```python
from build123d import *

# Parameters (mm, degrees)
F0_W     = 34
F0_H     = 10
F1_DEPTH = 5


with BuildPart() as f1:
    # F0 (on Top) → F1 (new body)
    with BuildSketch(Plane.XY):
        with Locations((5, 0)):
            Rectangle(F0_W, F0_H)
        with BuildLine():
            ThreePointArc((-9.081139, -2.25), (-8.767748, 2.440352), (-4.75, 0))
            ThreePointArc((-4.75, 0), (-5.059648, -1.267748), (-5.918861, -2.25))
            ThreePointArc((-5.918861, -2.25), (-7.5, -2.75), (-9.081139, -2.25))
        make_face(mode=Mode.SUBTRACT)
        Polygon((-3.175426, 0), (-1.587713, 2.75), (1.587713, 2.75), (3.175426, 0), (1.587713, -2.75), (-1.587713, -2.75), align=None, mode=Mode.SUBTRACT)
        Polygon((5.247223, 0), (7.123612, 3.25), (10.876388, 3.25), (12.752777, 0), (10.876388, -3.25), (7.123612, -3.25), align=None, mode=Mode.SUBTRACT)
        Polygon((20.098076, 0), (18.799038, -2.25), (16.200962, -2.25), (14.901924, 0), (16.200962, 2.25), (18.799038, 2.25), align=None, mode=Mode.SUBTRACT)
        with BuildLine():
            Line((-5.918861, -2.25), (-9.081139, -2.25))
            ThreePointArc((-9.081139, -2.25), (-7.5, -2.75), (-5.918861, -2.25))
        make_face()
    extrude(amount=F1_DEPTH)


solid = f1.part
```
The model under review builds one solid part; all positions refer to its coordinate system, in mm. A direction names the side the tool comes from. Give positions to 0.01 mm unless a question says otherwise; leave off trailing zeros. Loops run counter-clockwise (first coordinate to the right, second up) from the corner with the lowest first, then second, coordinate; pieces in that order, holes last. Notation, with made-up numbers: (-5.75, 24.25) -> (52.25, 24.25) arc R16 ccw to (52.25, 36.25) -> close; hole circle Ø1 at (45.25, 14). An arc over 180 degrees is marked (long way). Use CSV: the item, a comma, the result in double quotes.
1. Consider section A-A, the plane x = -7.5. Write out the cut boundary in (y, z), then the cut area to 3 significant figures.
Result:
outline,"(-5, 0) -> (-2.25, 0) -> (-2.25, 5) -> (-5, 5) -> close; (2.75, 0) -> (5, 0) -> (5, 5) -> (2.75, 5) -> close"
area,"25.0 mm²"
2. Consider section D-D, the plane x = 1. Write out the cut boundary in (y, z).
Result:
outline,"(-5, 0) -> (-2.75, 0) -> (-2.75, 5) -> (-5, 5) -> close; (2.75, 0) -> (5, 0) -> (5, 5) -> (2.75, 5) -> close"
3. For P1, Ø2, axis at x = 9.5, y = 1.5, coming from the -Z side, flat-tipped, find the tip position at first contact; note if it passes through.
Result:
P1,"passes through"
4. To check wall thickness, follow probe 1 along Y at (x, z) = (9, 1.1); probe 2 along Y at (x, z) = (-7.5, 3.95); probe 3 along X at (y, z) = (-2, 1.4). State the ranges of each line that lie inside material, in increasing order. Write a range as from..to.
Result:
probe 1,"y = -5..-3.25, 3.25..5"
probe 2,"y = -5..-2.25, 2.75..5"
probe 3,"x = -12..-9.39, -5.61..-2.02, 2.02..6.4, 11.6..16.06, 18.94..22"
5. Consider section B-B, the plane z = 4.5. Write out the cut boundary in (x, y).
Result:
outline,"(-12, -5) -> (22, -5) -> (22, 5) -> (-12, 5) -> close; hole (-9.08, -2.25) -> (-5.92, -2.25) arc R2.75 ccw to (-4.75, 0) arc R2.75 ccw (long way) to start; hole (-3.18, 0) -> (-1.59, -2.75) -> (1.59, -2.75) -> (3.18, 0) -> (1.59, 2.75) -> (-1.59, 2.75) -> close; hole (5.25, 0) -> (7.12, -3.25) -> (10.88, -3.25) -> (12.75, 0) -> (10.88, 3.25) -> (7.12, 3.25) -> close; hole (14.9, 0) -> (16.2, -2.25) -> (18.8, -2.25) -> (20.1, 0) -> (18.8, 2.25) -> (16.2, 2.25) -> close"
6. Consider section C-C, the plane y = 1. Write out the cut boundary in (x, z), then the cut area to 3 significant figures.
Result:
outline,"(-12, 0) -> (-10.06, 0) -> (-10.06, 5) -> (-12, 5) -> close; (-4.94, 0) -> (-2.6, 0) -> (-2.6, 5) -> (-4.94, 5) -> close; (2.6, 0) -> (5.82, 0) -> (5.82, 5) -> (2.6, 5) -> close; (12.18, 0) -> (15.48, 0) -> (15.48, 5) -> (12.18, 5) -> close; (19.52, 0) -> (22, 0) -> (22, 5) -> (19.52, 5) -> close"
area,"66.4 mm²"
7. The part is to be moulded in two halves that separate along X. For faces 1 (the face through (11.8, 1.65, 2.46)), 2 (the face through (0, -2.75, 2)), 3 (the face through (5, 5, 2)), 4 (the face through (22, 0, 2)), say which applies: +X half, -X half, draft (parallel to the pull), parting line (faces both ways), or undercut.
Result:
face 1,"undercut"
face 2,"undercut"
face 3,"draft"
face 4,"+X half"
8. Machinability: for faces 5 (the face through (5, 0, 5)), 6 (the face through (-7, -2.25, 2)), which of the approach directions +Z, -Z, +X, -X, +Y, -Y give a long, thin tool a straight path to every point of the face, cutting with its end or side? Answer none if there is none.
Result:
face 5,"+Z, +X, -X, +Y, -Y"
face 6,"+Z, -Z"
